Part model, mm, in its own coordinate system. A direction names the side the tool comes from. Coordinates: 2 decimals unless noted, no trailing zeros. Order: outer loops, then holes, each group sorted by start corner. A loop starts at its lowest first (then second) coordinate and runs counter-clockwise, first axis right, second up.
Autodesk Inventor part; units mm, degrees
ref_plane "YZ Plane" through (0, 0, 0) normal (1, 0, 0) x (0, 1, 0)
ref_plane "XZ Plane" through (0, 0, 0) normal (0, 1, 0) x (-1, 0, 0)
ref_plane "XY Plane" through (0, 0, 0) normal (0, 0, 1) x (1, 0, 0)
sketch "Skizze1" plane through (0, 0, 0) normal (0, 1, 0) x (-1, 0, 0)
  line L0 (4.5, 4) -> (-4.5, 4)
  line L1 (-4.5, 4) -> (-4.5, -4)
  line L2 (-4.5, -4) -> (4.5, -4)
  line L3 (4.5, -4) -> (4.5, 4)
  line L4 (4.5, 4) -> (-4.5, -4) construction
  line L5 (-4.5, 4) -> (4.5, -4) construction
  point P0 (0, 0)
  dimension "d0" = 9
  dimension "d1" = 8
extrude "Extrusion1" add sketch "Skizze1" along normal blind 3.5
fillet "Rundung1" radius 1 4 edges at (0, 3.5, 4) (0, 0, 4) (0, 3.5, -4) (0, 0, -4)
sketch "Skizze2" plane through (-4.5, 0, -3) normal (-1, 0, 0) x (0, 0, 1)
  line L0 (-1, 1) -> (-1, 2.5)
  arc A0 (0, 3.5) -> (-1, 2.5) centre (0, 2.5) ccw
  line L1 (0, 3.5) -> (6, 3.5)
  arc A1 (7, 2.5) -> (6, 3.5) centre (6, 2.5) ccw
  line L2 (7, 1) -> (7, 2.5)
  arc A2 (6, 0) -> (7, 1) centre (6, 1) ccw
  line L3 (0, 0) -> (6, 0)
  arc A3 (-1, 1) -> (0, 0) centre (0, 1) ccw
  line L4 (0.5, 2.5) -> (5.5, 2.5)
  line L5 (6, 2) -> (6, 1.5)
  line L6 (5.5, 1) -> (0.5, 1)
  line L7 (0, 1.5) -> (0, 2)
  arc A4 (0.5, 2.5) -> (0, 2) centre (0.5, 2) ccw
  arc A5 (0, 1.5) -> (0.5, 1) centre (0.5, 1.5) ccw
  arc A6 (5.5, 1) -> (6, 1.5) centre (5.5, 1.5) ccw
  arc A7 (6, 2) -> (5.5, 2.5) centre (5.5, 2) ccw
  line L8 (0, 3.1) -> (6, 3.1)
  line L9 (0, 0.4) -> (6, 0.4)
  line L10 (-0.6, 2.5) -> (-0.6, 1)
  line L11 (6.6, 2.5) -> (6.6, 1)
  arc A8 (0, 3.1) -> (-0.6, 2.5) centre (0, 2.5) ccw
  arc A9 (6.6, 2.5) -> (6, 3.1) centre (6, 2.5) ccw
  arc A10 (6, 0.4) -> (6.6, 1) centre (6, 1) ccw
  arc A11 (-0.6, 1) -> (0, 0.4) centre (0, 1) ccw
  point P0 (3, 0)
  dimension "d5" = 0.5
  dimension "d6" = 0.4
  dimension "d7" = 0.4
  dimension "d8" = 0.4
  dimension "d9" = 0.4
extrude "Extrusion2" cut sketch "Skizze2" against normal blind 5 contours L8 A9 L11 A10 L9 A11 L10 A8
sketch "Skizze3" plane through (0, 0, 0) normal (0, -1, 0) x (1, 0, 0)
  line L0 (-4.5, 3) -> (4.5, 3)
  line L1 (4.5, 4) -> (-4.5, 4)
  line L2 (-2.5, 3) -> (0.5, 3)
  line L3 (0.5, 3) -> (0.5, 4)
  line L4 (0.5, 4) -> (-2.5, 4)
  line L5 (-2.5, 4) -> (-2.5, 3)
  line L6 (-4.5, 3) -> (-4.5, 4)
  line L7 (-2.8823, 0) -> (1.7829, 0)
  line L8 (-4.5, -3) -> (4.5, -3)
  line L9 (4.5, -4) -> (-4.5, -4)
  line L10 (0.5, -3) -> (0.5, -4)
  line L11 (-2.5, -4) -> (-2.5, -3)
  point P0 (0, 0)
  dimension "d12" = 2
  dimension "d13" = 3
extrude "Extrusion3" add sketch "Skizze3" against normal blind 1 contours L5 L1 L3 L0 | L8 L10 L9 L11
properties part number "USB-C"
(1) Tool access for faces 4 (the face through (0.5, 0.16, 3.79)), 5 (the face through (-3.486, 0.301, 3.715)), 6 (the face through (0.5, 0.16, -3.79)), 7 (the face through (-2, 3.1, 0)), 8 (the face through (0, 2, -4)): list every direction of +Z, -Z, +X, -X, +Y, -Y with a clear straight run to the whole face (end or side of a thin tool).
(2) Slice it at A-A, the plane x = 0. Give the cut face in (y, z).
(3) Pull direction Y, two halves, no side cores. Call faces 1 (the face through (-0.063, 3.215, -3.699)), 2 (the face through (-4.5, 2, 0)), 3 (the face through (-2, 0.4, 0)): +Y half, -Y half, draft (parallel to the pull), parting line (faces both ways), or undercut.
(4) Slice it at B-B, the plane y = 1.65. Give the cut face in (x, z).
(5) Slice it at D-D, the plane z = -2.75. Give the cut face in (x, y), then the cut area to 3 significant figures.
(6) Probe line 1 (Y direction, x = -3.25, z = 1.5); line 2 (Z direction, x = -1.25, y = 2.4); line 3 (X direction, y = 1.45, z = 3.25). List the from-to ranges inside material, lowest first.
(7) Slice it at C-C, the plane x = 1. Give the cut face in (y, z).
(8) Drop a flat-ended pin along its axis: pin 1 (0.5 mm diameter, centred on x = -0.5, z = -3.5, fed in from +Y). Give the stop position or say it passes through.
Here are the results:
1. face 4: +Z, +X, -Y
1. face 5: +Z, -X, -Y
1. face 6: -Z, +X, -Y
1. face 7: -X
1. face 8: -Z, +X, -X, +Y, -Y
2. outline: (0, -4) - (2.5, -4) arc R1 ccw to (3.5, -3) - (3.5, 3) arc R1 ccw to (2.5, 4) - (0, 4) - close; (1, -2.5) arc R0.5 ccw to (1.5, -3) - (2, -3) arc R0.5 ccw to (2.5, -2.5) - (2.5, 2.5) arc R0.5 ccw to (2, 3) - (1.5, 3) arc R0.5 ccw to (1, 2.5) - close; hole (0.4, -3) - (1, -3) - (1, -3.6) - (2.5, -3.6) arc R0.6 ccw to (3.1, -3) - (3.1, 3) arc R0.6 ccw to (2.5, 3.6) - (1, 3.6) - (1, 3) - (0.4, 3) - close
3. face 1: +Y half
3. face 2: draft
3. face 3: undercut
4. outline: (-4.5, -4) - (4.5, -4) - (4.5, 4) - (-4.5, 4) - (-4.5, 3.6) - (0.5, 3.6) - (0.5, 3) - (-4.5, 3) - (-4.5, -3) - (0.5, -3) - (0.5, -3.6) - (-4.5, -3.6) - close
5. outline: (-4.5, 0) - (4.5, 0) - (4.5, 3.5) - (-4.5, 3.5) - (-4.5, 3.1) - (0.5, 3.1) - (0.5, 2.43) - (-4.5, 2.43) - (-4.5, 1.07) - (0.5, 1.07) - (0.5, 0.4) - (-4.5, 0.4) - close
5. area: 24.8 mm2
6. line 1: y = 0 to 0.4, 1 to 2.5, 3.1 to 3.5
6. line 2: z = -4 to -3.6, -2.8 to 2.8, 3.6 to 4
6. line 3: x = 0.5 to 4.5
7. outline: (0, -3) arc R1 ccw to (1, -4) - (2.5, -4) arc R1 ccw to (3.5, -3) - (3.5, 3) arc R1 ccw to (2.5, 4) - (1, 4) arc R1 ccw to (0, 3) - close
8. pin 1: stops at y = 3.47
